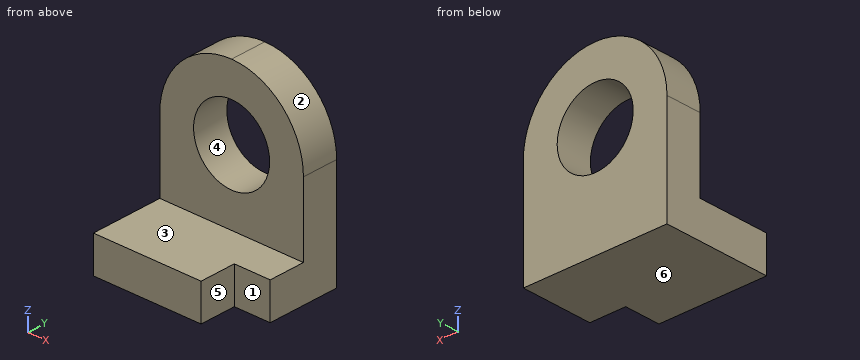
from build123d import *

# Parameters (mm, degrees)
F0_W     = 101.6
F0_H     = 76.2
F1_DEPTH = 25.4
F2_W     = 25.4
F2_H     = 25.4
F3_DEPTH = 25.401
F4_W     = 101.6
F4_H     = 25.4
F5_DEPTH = 101.6
F6_R     = 50.8
F7_R     = 50.79999
F8_R     = 26.8874983084
F9_DEPTH = 25.401


# Not quite as in the source:
# - a fillet or chamfer is up to 0.001 mm smaller than in the source, because OpenCascade refuses the exact size


with BuildPart() as f1:
    # F0 (on Top) → F1 (new body)
    with BuildSketch(Plane.XY):
        Rectangle(F0_W, F0_H)
    extrude(amount=F1_DEPTH)

    # F2 (on face) → F3 (cut, through all)
    with BuildSketch(Plane.XY.offset(25.4)):
        with Locations((38.1, -25.4)):
            Rectangle(F2_W, F2_H)
    extrude(amount=-F3_DEPTH, mode=Mode.SUBTRACT)

    # F4 (on face) → F5 (join)
    with BuildSketch(Plane.XY.offset(25.4)):
        with Locations((0, 25.4)):
            Rectangle(F4_W, F4_H)
    extrude(amount=F5_DEPTH)

    # F6
    f6_edges = [f1.edges().sort_by_distance(p)[0] for p in [
        (-50.8, 25.4, 127),
    ]]
    fillet(f6_edges, radius=F6_R)

    # F7 (radius 50.8 in the source; OpenCascade refuses exactly that, so slightly less here)
    f7_edges = [f1.edges().sort_by_distance(p)[0] for p in [
        (50.8, 25.4, 127),
    ]]
    fillet(f7_edges, radius=F7_R)

    # F8 (on face) → F9 (cut, through all)
    with BuildSketch(Plane.XZ.offset(-12.7)):
        with Locations((0, 76.2)):
            Circle(F8_R)
    extrude(amount=-F9_DEPTH, mode=Mode.SUBTRACT)


solid = f1.part
Read the model definition and answer for the solid it produces. Units are mm, in the model's axes. Face numbers are marked on the shaded views. A direction names the side the tool comes from. Coordinates: 2 decimals unless noted, no trailing zeros. Order: outer loops, then holes, each group sorted by start corner. A loop starts at its lowest first (then second) coordinate and runs counter-clockwise, first axis right, second up. Notation, with made-up numbers: M 38.25,-2.5 L 84.25,-2.5 A32 ccw 84.25,27.5 Z; hole C -25.75,66 d6. An arc over 180 degrees is marked long. Put each result on its own line as item: value. Start each with the question number.
Item 1: For the marked faces 1, 2 and 3, determine the directions among +Z, -Z, +X, -X, +Y, -Y from which every point of the face is accessible in a straight line to the end or side of a thin tool.
Item 2: Section C-C, the plane y = -4 is taken. Determine the outline of the cut face in (x, z).
Item 3: Section D-D, the plane x = 38 is taken. Determine the outline of the cut face in (y, z).
Item 4: Consider probe 1 along X at (y, z) = (19, 76); probe 2 along Z at (x, y) = (-28, -30.5); probe 3 along X at (y, z) = (17.5, 99). Determine where each line is inside the solid, lowest interval first. Write a range as [from, to].
Item 5: Section B-B, the plane x = 23 is taken. Determine the outline of the cut face in (y, z), plus the area to 3 significant figures.
Item 6: Given pin 1 Ø6 at (y, z) = (20, 99) entering from +X; pin 2 Ø3 at (x, z) = (40, 43.5) entering from -Y, each flat-ended and moving along its own axis, determine where each tip first touches the part or whether it passes through.
Item 7: Section A-A, the plane z = 69.5 is taken. Determine the outline of the cut face in (x, y).
Item 8: The mould has two halves that part along X. Classify the marked faces 4, 5 and 6: +X half, -X half, draft (parallel to the pull), parting line (faces both ways), or undercut.
Computed:
1. face 1: +Z, -Z, +X, -Y
1. face 2: +Z, +X, +Y, -Y
1. face 3: +Z, +X, -X, -Y
2. outline: M -50.8,0 L 50.8,0 L 50.8,25.4 L -50.8,25.4 Z
3. outline: M -12.7,0 L 38.1,0 L 38.1,109.91 L 12.7,109.91 L 12.7,25.4 L -12.7,25.4 Z
4. probe 1: x = [-50.8, -26.89], [26.89, 50.8]
4. probe 2: z = [0, 25.4]
4. probe 3: x = [-45.4, -14.25], [14.25, 45.4]
5. outline: M -38.1,0 L 38.1,0 L 38.1,62.27 L 12.7,62.27 L 12.7,25.4 L -38.1,25.4 Z; M 12.7,90.13 L 38.1,90.13 L 38.1,121.5 L 12.7,121.5 Z
5. area: 3,670 mm2
6. pin 1: stops at x = 46.78
6. pin 2: stops at y = 12.7
7. outline: M -50.8,12.7 L -26.04,12.7 L -26.04,38.1 L -50.8,38.1 Z; M 26.04,12.7 L 50.8,12.7 L 50.8,38.1 L 26.04,38.1 Z
8. face 4: undercut
8. face 5: +X half
8. face 6: draft
